Autodesk Inventor part; units mm, degrees
ref_plane "YZ Plane" through (0, 0, 0) normal (1, 0, 0) x (0, 1, 0)
ref_plane "XZ Plane" through (0, 0, 0) normal (0, 1, 0) x (-1, 0, 0)
ref_plane "XY Plane" through (0, 0, 0) normal (0, 0, 1) x (1, 0, 0)
sketch "Sketch5" plane through (0, 0, 0) normal (0, 1, 0) x (-1, 0, 0)
  circle A0 centre (0, 0) radius 50
  dimension "d10" = 100
extrude "Extrusion4" add sketch "Sketch5" along normal blind 5
sketch "Sketch6" plane through (0, 5, 0) normal (0, 1, 0) x (1, 0, 0)
  circle A0 centre (0, 0) radius 6.25
  dimension "d13" = 12.5
extrude "Extrusion5" cut sketch "Sketch6" against normal blind 5
sketch "Sketch7" plane through (0, 5, 0) normal (0, 1, 0) x (1, 0, 0)
  circle A0 centre (0, 0) radius 50 construction
  line L0 (9.75, 0) -> (4.875, -8.4437)
  line L1 (4.875, -8.4437) -> (-4.875, -8.4437)
  line L2 (-4.875, -8.4437) -> (-9.75, 0)
  line L3 (-9.75, 0) -> (-4.875, 8.4437)
  line L4 (-4.875, 8.4437) -> (4.875, 8.4437)
  line L5 (4.875, 8.4437) -> (9.75, 0)
  line L6 (0, 0) -> (50, 0) construction
  circle A1 centre (0, 0) radius 15
  dimension "d20" = 19.5
  dimension "d21" = 30
extrude "Extrusion6" add sketch "Sketch7" along normal blind 10
sketch "Sketch8" plane through (0, 15, 0) normal (0, 1, 0) x (1, 0, 0)
  circle A0 centre (0, 0) radius 12.5 construction
  line L0 (0, 12.5) -> (0, -12.5) construction
  line L1 (-12.5, 0) -> (12.5, 0) construction
  circle A1 centre (0, 12.5) radius 1.75
  circle A2 centre (-12.5, 0) radius 1.75
  circle A3 centre (0, -12.5) radius 1.75
  circle A4 centre (12.5, 0) radius 1.75
  dimension "d24" = 25
  dimension "d25" = 3.5
  dimension "d26" = 3.5
  dimension "d27" = 3.5
  dimension "d28" = 3.5
extrude "Extrusion7" cut sketch "Sketch8" against normal blind 5
sketch "Sketch9" plane through (0, 5, 0) normal (0, 1, 0) x (1, 0, 0)
  circle A0 centre (0, 0) radius 50
  circle A1 centre (0, 0) radius 47.5
  dimension "d31" = 95
extrude "Extrusion8" add sketch "Sketch9" along normal blind 30
sketch "Sketch10" plane through (0, 5, 0) normal (0, 1, 0) x (1, 0, 0)
  circle A0 centre (0, 0) radius 40 construction
  line L0 (40, 0) -> (-40, 0) construction
  line L1 (0, 40) -> (0, -40) construction
  circle A1 centre (40, 0) radius 4.5
  circle A2 centre (0, 40) radius 4.5
  circle A3 centre (0, -40) radius 4.5
  circle A4 centre (-40, 0) radius 4.5
  dimension "d34" = 80
  dimension "d35" = 9
  dimension "d36" = 9
  dimension "d37" = 9
  dimension "d38" = 9
extrude "Extrusion9" add sketch "Sketch10" along normal blind 30
sketch "Sketch11" plane through (40, 35, 0) normal (0, 1, 0) x (1, 0, 0)
  circle A0 centre (0, 0) radius 2.5
  point P0 (-40, 0)
  dimension "d41" = 5
extrude "Extrusion10" cut sketch "Sketch11" against normal blind 20
sketch "Sketch12" plane through (0, 35, -40) normal (0, 1, 0) x (1, 0, 0)
  circle A0 centre (0, 0) radius 2.5
  point P0 (0, -40)
  dimension "d44" = 5
extrude "Extrusion11" cut sketch "Sketch12" against normal blind 20
sketch "Sketch13" plane through (-40, 35, 0) normal (0, 1, 0) x (1, 0, 0)
  circle A0 centre (0, 0) radius 2.5
  point P0 (40, 0)
  dimension "d47" = 5
extrude "Extrusion12" cut sketch "Sketch13" against normal blind 20
sketch "Sketch14" plane through (0, 35, 40) normal (0, 1, 0) x (1, 0, 0)
  circle A0 centre (0, 0) radius 2.5
  point P0 (0, 40)
  dimension "d50" = 5
extrude "Extrusion13" cut sketch "Sketch14" against normal blind 20
sketch "Sketch16" plane through (0, 5, 0) normal (0, 1, 0) x (1, 0, 0)
  circle A0 centre (0, 0) radius 47.5 construction
  line L0 (0, 47.5) -> (0, -47.5) construction
  line L1 (-47.5, 0) -> (47.5, 0) construction
  circle A1 centre (-40, 0) radius 2.5 construction
  circle A2 centre (-40, 0) radius 4.5 construction
  circle A3 centre (-40, 0) radius 4.5 construction
  line L2 (-40, 4.5) -> (-40, -4.5) construction
  circle A4 centre (0, 0) radius 47.5 construction
  line L3 (-40, 4.5) -> (-46.2643, 10.7643)
  line L4 (-40, 4.5) -> (-31.141, 4.5) construction
  line L5 (-40, -4.5) -> (-46.2643, -10.7643)
  arc A5 (-46.2643, 10.7643) -> (-46.2643, -10.7643) centre (0, 0) ccw
  arc A6 (-40, 4.5) -> (-40, -4.5) centre (-40, 0) ccw
  circle A7 centre (0, 0) radius 47.5 construction
  circle A8 centre (40, 0) radius 4.5 construction
  circle A9 centre (0, 0) radius 47.5 construction
  line L6 (40, 4.5) -> (46.2643, 10.7643)
  line L7 (40, -4.5) -> (46.2643, -10.7643)
  arc A10 (46.2643, -10.7643) -> (46.2643, 10.7643) centre (0, 0) ccw
  arc A11 (40, -4.5) -> (40, 4.5) centre (40, 0) ccw
  circle A12 centre (0, -40) radius 2.5 construction
  circle A13 centre (0, -40) radius 4.5 construction
  circle A14 centre (0, -40) radius 4.5 construction
  line L8 (4.5, -40) -> (-4.5, -40) construction
  line L9 (-4.5, -40) -> (-10.7643, -46.2643)
  line L10 (4.5, -40) -> (10.7643, -46.2643)
  arc A15 (-10.7643, -46.2643) -> (10.7643, -46.2643) centre (0, 0) ccw
  arc A16 (-4.5, -40) -> (4.5, -40) centre (0, -40) ccw
  line L11 (-4.5, 40) -> (-10.7643, 46.2643)
  line L12 (4.5, 40) -> (10.7643, 46.2643)
  arc A17 (10.7643, 46.2643) -> (-10.7643, 46.2643) centre (0, 0) ccw
  arc A18 (4.5, 40) -> (-4.5, 40) centre (0, 40) ccw
  dimension "d54" = 135
extrude "Extrusion14" add sketch "Sketch16" along normal blind 30
chamfer "Chamfer1" distance 1 angle 45 1 edges at (-50, 35, 0)
chamfer "Chamfer2" distance 2 angle 45 1 edges at (50, 0, 0)
properties part number "ground_support_0"
Could you check a few things on this model? Use its own coordinates, in mm. A direction names the side the tool comes from. Coordinates: 2 decimals unless noted, no trailing zeros. Loops run counter-clockwise (first coordinate to the right, second up) from the corner with the lowest first, then second, coordinate; pieces in that order, holes last.
1. We'd pull the mould along X, two halves only. Please class faces 3 (the face through (-7.28, 9.93, 4.28)), 4 (the face through (-10, 0, 1)), 5 (the face through (-44.46, 0.13, -18.43)), 6 (the face through (7.6, 19.8, -43.1)): released by +X, released by -X, zero draft, split by the parting line, or undercut.
2. Imagine slicing it at A-A (y = 32). Please give me the cut outline in (x, z), and give its area (3 significant figures).
3. I need wall thicknesses on L1, parallel to X at y = 20, z = 0; L2, parallel to Z at x = 0, y = 12.6; L3, parallel to X at y = 13, z = 0. Which ranges of each line are inside material? Lowest first, please.
4. For faces 1 (the face through (0, 35, 36)), 2 (the face through (-40, 15, 0)), which set-ups out of +Z, -Z, +X, -X, +Y, -Y let a thin tool reach every point of the face, with its end or its side?
5. For P1, Ø4, axis at x = -15, y = 14.5, coming from the -Z side; P2, Ø8, axis at y = 12.5, z = 13.5, coming from the +X side; P3, Ø10.5, axis at x = 1.5, y = 10, coming from the +Z side, each with a flat end and sliding along its axis, tell me the tip position at first contact or that it passes through.
Computed values:
1. face 3: undercut
1. face 4: zero draft
1. face 5: split by the parting line
1. face 6: undercut
2. outline: circle Ø100 at (0, 0); hole (-46.26, -10.76) arc R47.5 ccw to (-10.76, -46.26) - (-4.5, -40) arc R4.5 cw to (4.5, -40) - (10.76, -46.26) arc R47.5 ccw to (46.26, -10.76) - (40, -4.5) arc R4.5 cw to (40, 4.5) - (46.26, 10.76) arc R47.5 ccw to (10.76, 46.26) - (4.5, 40) arc R4.5 cw to (-4.5, 40) - (-10.76, 46.26) arc R47.5 ccw to (-46.26, 10.76) - (-40, 4.5) arc R4.5 cw to (-40, -4.5) - close; hole circle Ø5 at (-40, 0); hole circle Ø5 at (0, -40); hole circle Ø5 at (0, 40); hole circle Ø5 at (40, 0)
2. area: 1,270 mm2
3. L1: x = -50 to -42.5, -37.5 to -35.5, 35.5 to 37.5, 42.5 to 50
3. L2: z = -50 to -35.5, -15 to -14.25, -10.75 to -8.44, 8.44 to 10.75, 14.25 to 15, 35.5 to 50
3. L3: x = -50 to -35.5, -15 to -14.25, -10.75 to -9.75, 9.75 to 10.75, 14.25 to 15, 35.5 to 50
4. face 1: +Z, -Z, +X, -X, +Y
4. face 2: +Y
5. P1: stops at z = -48.28
5. P2: stops at x = 49.09
5. P3: stops at z = 50
